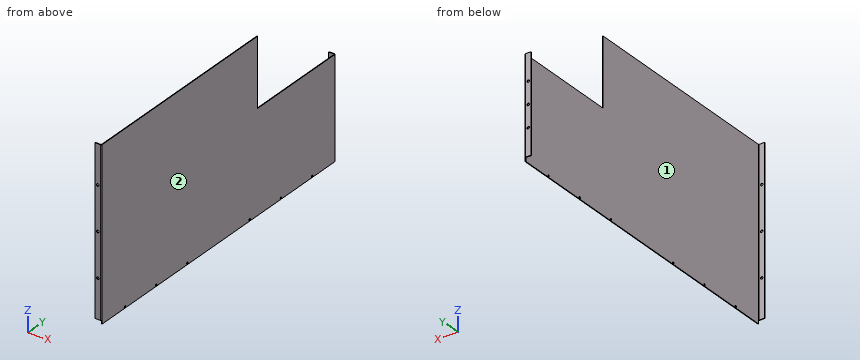
```python
from build123d import *

# Parameters (mm, degrees)
SKETCH_1_W                       = 1.5
SKETCH_1_H                       = 750
SM_BASE_FLANGE_1_DEPTH           = 385
SM_EDGE_FLANGE_1_STRIP_W         = 7.4732
SM_EDGE_FLANGE_1_STRIP_H         = 1.5
SM_EDGE_FLANGE_1_STRIP_CUT_DEPTH = 385
SM_EDGE_FLANGE_1_DEPTH           = 385
SM_EDGE_FLANGE_2_STRIP_W         = 7.4732
SM_EDGE_FLANGE_2_STRIP_H         = 1.5
SM_EDGE_FLANGE_2_STRIP_CUT_DEPTH = 385
SM_EDGE_FLANGE_2_DEPTH           = 385
SKETCH_12_W                      = 17.104155355
SKETCH_12_H                      = 8.497904819
CUT_EXTRUDE_1_DEPTH              = 8
CUT_EXTRUDE_START                = -8
CUT_EXTRUDE_3_DEPTH              = 8
SKETCH_16_W                      = 51.042433358
SKETCH_16_H                      = 155
CUT_EXTRUDE_4_DEPTH              = 248.5
SKETCH_17_R                      = 2.75
CUT_EXTRUDE_5_DEPTH              = 20
SKETCH_18_R                      = 2.75
CUT_EXTRUDE_6_DEPTH              = 20
SKETCH_19_W                      = 1.5
SKETCH_19_H                      = 155
CUT_EXTRUDE_7_DEPTH              = 1.5
SKETCH_21_R                      = 2.25
CUT_EXTRUDE_9_DEPTH              = 10


# Read off the part's stored shape, not the designer's step: 切除-拉伸3
# Sheet-metal steps are written as plain solids
with BuildPart() as part:
    # Sketch 1 → 基体-法兰1 (new body)
    with BuildSketch(Plane.XY):
        with Locations((0.75, 375)):
            Rectangle(SKETCH_1_W, SKETCH_1_H)
    extrude(amount=SM_BASE_FLANGE_1_DEPTH)

    # 边线-法兰1 strip (across the edge) → 边线-法兰1 strip cut (cut)
    with BuildSketch(Plane(origin=(0, 750, 385), x_dir=(0, -1, 0), z_dir=(0, 0, -1))):
        with Locations((-1.5, -0.75)):
            Rectangle(SM_EDGE_FLANGE_1_STRIP_W, SM_EDGE_FLANGE_1_STRIP_H)
    extrude(amount=SM_EDGE_FLANGE_1_STRIP_CUT_DEPTH, mode=Mode.SUBTRACT)

    # 边线-法兰1 section (across the edge) → 边线-法兰1 (add)
    with BuildSketch(Plane(origin=(0, 750, 385), x_dir=(0, -1, 0), z_dir=(0, 0, -1))):
        with BuildLine():
            Line((0, 0.7366), (0, 13.5))
            Line((0, 13.5), (1.5, 13.5))
            Line((1.5, 13.5), (1.5, 0.7366))
            ThreePointArc((1.5, 0.7366), (1.715745145, 0.215745145), (2.2366, 0))
            Line((2.2366, 0), (2.2366, -1.5))
            ThreePointArc((2.2366, -1.5), (0.655084973, -0.844915027), (0, 0.7366))
        make_face()
    extrude(amount=SM_EDGE_FLANGE_1_DEPTH)

    # 边线-法兰2 strip (across the edge) → 边线-法兰2 strip cut (cut)
    with BuildSketch(Plane(origin=(0, 0, 0), x_dir=(0, 1, 0), z_dir=(0, 0, 1))):
        with Locations((-1.5, -0.75)):
            Rectangle(SM_EDGE_FLANGE_2_STRIP_W, SM_EDGE_FLANGE_2_STRIP_H)
    extrude(amount=SM_EDGE_FLANGE_2_STRIP_CUT_DEPTH, mode=Mode.SUBTRACT)

    # 边线-法兰2 section (across the edge) → 边线-法兰2 (add)
    with BuildSketch(Plane(origin=(0, 0, 0), x_dir=(0, 1, 0), z_dir=(0, 0, 1))):
        with BuildLine():
            Line((0, 0.7366), (0, 13.5))
            Line((0, 13.5), (1.5, 13.5))
            Line((1.5, 13.5), (1.5, 0.7366))
            ThreePointArc((1.5, 0.7366), (1.715745145, 0.215745145), (2.2366, 0))
            Line((2.2366, 0), (2.2366, -1.5))
            ThreePointArc((2.2366, -1.5), (0.655084973, -0.844915027), (0, 0.7366))
        make_face()
    extrude(amount=SM_EDGE_FLANGE_2_DEPTH)

    # 草图12 → 切除-拉伸1 (cut)
    with BuildSketch(Plane(origin=(0, 0, 0), x_dir=(-1, 0, 0), z_dir=(0, 0, -1))):
        with Locations((7.052077678, 752.01235241)):
            Rectangle(SKETCH_12_W, SKETCH_12_H)
    extrude(amount=-CUT_EXTRUDE_1_DEPTH, mode=Mode.SUBTRACT)

    # 切除-拉伸3 outline → 切除-拉伸3 (cut)
    with BuildSketch(Plane(origin=(0, 0, 0), x_dir=(-1, 0, 0), z_dir=(0, 0, -1)).offset(CUT_EXTRUDE_START)):
        with BuildLine():
            Line((0, 2.2366), (-1.5, 2.2366))
            ThreePointArc((-1.5, 2.2366), (-0.844915027, 0.655084973), (0.7366, 0))
            Line((0.7366, 0), (13.5, 0))
            Line((13.5, 0), (13.5, 1.5))
            Line((13.5, 1.5), (0.7366, 1.5))
            ThreePointArc((0.7366, 1.5), (0.215745145, 1.715745145), (0, 2.2366))
        make_face()
    extrude(amount=CUT_EXTRUDE_3_DEPTH, mode=Mode.SUBTRACT)

    # 草图16 → 切除-拉伸4 (cut)
    with BuildSketch(Plane(origin=(0, 750, 0), x_dir=(1, 0, 0), z_dir=(0, 1, 0))):
        with Locations((12.021216679, -307.5)):
            Rectangle(SKETCH_16_W, SKETCH_16_H)
    extrude(amount=-CUT_EXTRUDE_4_DEPTH, mode=Mode.SUBTRACT)

    # 草图17 → 切除-拉伸5 (cut)
    with BuildSketch(Plane(origin=(0, 1.5, 0), x_dir=(1, 0, 0), z_dir=(0, 1, 0))):
        with Locations(Location((-7.1183, -296.5, 0), (0, 0, 180))):
            Circle(SKETCH_17_R)
        with Locations(Location((-7.1183, -196.5, 0), (0, 0, 180))):
            Circle(SKETCH_17_R)
        with Locations((-7.1183, -96.5)):
            Circle(SKETCH_17_R)
    extrude(amount=-CUT_EXTRUDE_5_DEPTH, mode=Mode.SUBTRACT)

    # 草图18 → 切除-拉伸6 (cut)
    with BuildSketch(Plane.XZ.offset(-748.5)):
        with Locations(Location((-7.1183, 69, 0), (0, 0, 270))):
            Circle(SKETCH_18_R)
        with Locations(Location((-7.1183, 119, 0), (0, 0, 270))):
            Circle(SKETCH_18_R)
        with Locations(Location((-7.1183, 169, 0), (0, 0, 270))):
            Circle(SKETCH_18_R)
    extrude(amount=-CUT_EXTRUDE_6_DEPTH, mode=Mode.SUBTRACT)

    # 草图19 → 切除-拉伸7 (cut)
    with BuildSketch(Plane(origin=(0, 501.5, 0), x_dir=(1, 0, 0), z_dir=(0, 1, 0))):
        with Locations((0.75, -307.5)):
            Rectangle(SKETCH_19_W, SKETCH_19_H)
    extrude(amount=-CUT_EXTRUDE_7_DEPTH, mode=Mode.SUBTRACT)

    # 草图21 → 切除-拉伸9 (cut)
    with BuildSketch(Plane(origin=(1.5, 0, 0), x_dir=(0, 0, -1), z_dir=(1, 0, 0))):
        with Locations((-3, 75)):
            Circle(SKETCH_21_R)
        with Locations((-3, 175)):
            Circle(SKETCH_21_R)
        with Locations((-3, 275)):
            Circle(SKETCH_21_R)
        with Locations(Location((-3, 475, 0), (0, 0, 180))):
            Circle(SKETCH_21_R)
        with Locations(Location((-3, 575, 0), (0, 0, 180))):
            Circle(SKETCH_21_R)
        with Locations(Location((-3, 675, 0), (0, 0, 180))):
            Circle(SKETCH_21_R)
    extrude(amount=-CUT_EXTRUDE_9_DEPTH, mode=Mode.SUBTRACT)


solid = part.part
```
Input: part model. Units: mm. Frame: model coordinates. Face numbers are marked on the shaded views. Round coordinates to 2 decimals unless told otherwise and drop trailing zeros. Loops run counter-clockwise (first coordinate to the right, second up) from the corner with the lowest first, then second, coordinate; pieces in that order, holes last. Notation, with made-up numbers: M -10,-8 L 12,-8 A7 cw 12,2 Z; hole C 44,19 d5. An arc over 180 degrees is marked long. Answer in a Markdown table with one row per item. Add a question column.
1. Mould query, pull axis Y, two halves, no side actions, for the marked faces 1 and 2. Classes: released by +Y, released by -Y, zero draft, split by the parting line, or undercut.
2. Section C-C (y = 647). Output: boundary loops of the cut face in (x, z), and give its area (3 significant figures).
3. Section A-A (z = 209.5). Output: boundary loops of the cut face in (x, y), and give its area (3 significant figures).
4. Ray query, probe 1 along Z at (x, y) = (1.15, 575); probe 2 along Y at (x, z) = (-12.25, 204.5); probe 3 along Z at (x, y) = (0.8, 275). Return the intervals inside material, ascending.
5. Contact query for flat-ended pins moving along their axis: pin 1 (1.6 mm diameter, centred on x = 0.5, z = 276.5, fed in from +Y); pin 2 (6 mm diameter, centred on y = 675, z = 3, fed in from -X); pin 3 (3.5 mm diameter, centred on x = -7.12, z = 196.5, fed in from -Y). Output: stop coordinate, or through.
6. Section B-B (y = 455.5). Output: boundary loops of the cut face in (x, z), and give its area (4 significant figures).
Values follow:
| question | item | result |
|---|---|---|
| 1 | face 1 | undercut |
| 1 | face 2 | zero draft |
| 2 | outline | M 0,0 L 1.5,0 L 1.5,230 L 0,230 Z |
| 2 | area | 345 mm^2 |
| 3 | outline | M -13.5,0 L -0.74,0 A2.24 ccw 1.5,2.24 L 1.5,747.76 A2.24 ccw -0.74,750 L -13.5,750 L -13.5,748.5 L -0.74,748.5 A0.74 cw 0,747.76 L 0,2.24 A0.74 cw -0.74,1.5 L -13.5,1.5 Z |
| 3 | area | 1,160 mm^2 |
| 4 | probe 1 | 0 to 0.75, 5.25 to 230 |
| 4 | probe 2 | 0 to 1.5, 748.5 to 750 |
| 4 | probe 3 | 0 to 0.75, 5.25 to 385 |
| 5 | pin 1 | y = 500 |
| 5 | pin 2 | x = 0 |
| 5 | pin 3 | y = 748.5 |
| 6 | outline | M 0,0 L 1.5,0 L 1.5,385 L 0,385 Z |
| 6 | area | 577.5 mm^2 |
